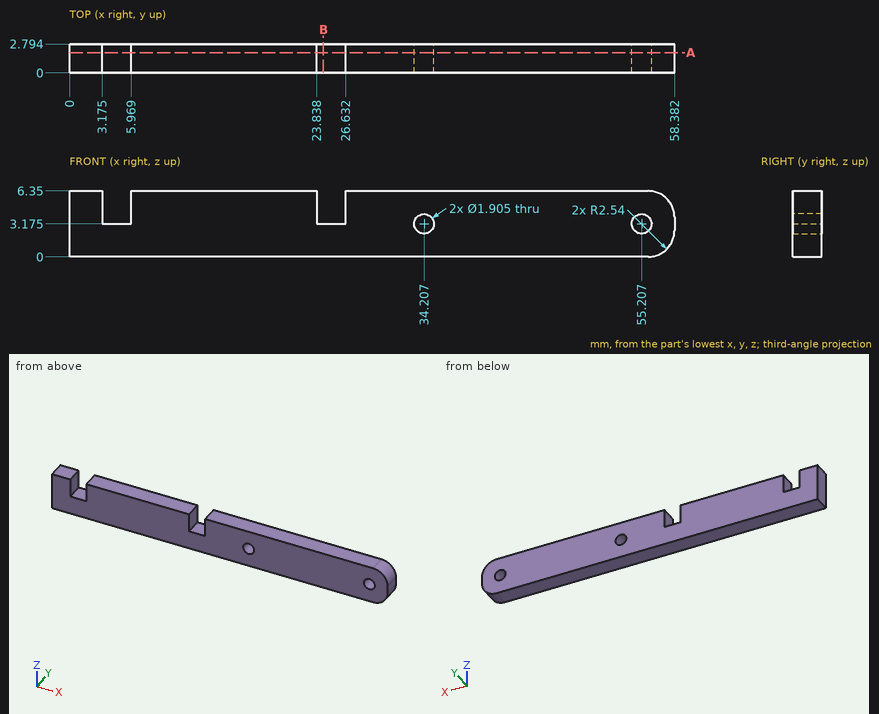
Study the drawing (mm; zero at the part's minimum x, y, z) and answer. Give positions to 0.01 mm unless a question says otherwise; leave off trailing zeros. Write each loop counter-clockwise with the first axis right and the second up, starting at its lowest first coordinate (ties: lowest second). Pieces come first, ordered by that corner, then holes. Notation, with made-up numbers: (30, 79) - (41, 79) arc R17 cw to (41, 109) - close; hole circle Ø11 at (-4, -4.75). An arc over 180 degrees is marked (long way). One line per question, with ' | ' between items. Start each with the question number.
1. Given P1, Ø1.1, axis at x = 55.21, z = 3.18, coming from the +Y side; P2, Ø1.4, axis at x = 4.5, y = 1.5, coming from the +Z side (3 decimals), each flat-ended and moving along its own axis, determine where each tip first touches the part or whether it passes through.
2. Straight lines are drawn through the part: line 1 (X direction, y = 0.7, z = 3.25) (1 decimal); line 2 (X direction, y = 2.05, z = 3.5) (1 decimal); line 3 (X direction, y = 2.35, z = 4.25) (1 decimal). For each, find the intervals that lie inside material, in ascending order.
3. Section A-A, the plane y = 1.95 is taken. Count the separate pieces of the cut face and the enclosed holes in it.
4. Section B-B, the plane x = 24.5 is taken. Determine the outline of the cut face in (y, z) (3 decimals), then the cut area to 3 significant figures.
Result:
1) P1: passes through | P2: stops at z = 3.175
2) line 1: x = 0 to 3.2, 6 to 23.8, 26.6 to 33.3, 35.2 to 54.3, 56.2 to 58.4 | line 2: x = 0 to 3.2, 6 to 23.8, 26.6 to 33.3, 35.1 to 54.3, 56.1 to 58.4 | line 3: x = 0 to 3.2, 6 to 23.8, 26.6 to 58.3
3) separate pieces: 1 | enclosed holes: 2
4) outline: (0, 0) - (2.794, 0) - (2.794, 3.175) - (0, 3.175) - close | area: 8.87 mm2
